from build123d import *

# Parameters (mm, degrees)
F0_W     = 90
F0_H     = 800
F1_DEPTH = 12
F3_D     = 15
F4_SIZE2 = 74.6410161514
F4_SIZE  = 20
F6_D     = 5


with BuildPart() as f1:
    # F0 (on Front) → F1 (new body)
    with BuildSketch(Plane.XZ):
        with Locations((45, -400)):
            Rectangle(F0_W, F0_H)
    extrude(amount=F1_DEPTH)

    # F3 (through all)
    with Locations(Plane.XZ.offset(12)):
        with Locations((45, -35)):
            Hole(F3_D / 2)

    # F4
    f4_edges = [f1.edges().sort_by_distance(p)[0] for p in [
        (90, -6, -800),
    ]]
    f4_side = f1.faces().sort_by_distance((90, -6, -400))[0]
    chamfer(f4_edges, length=F4_SIZE, length2=F4_SIZE2, reference=f4_side)

    # F6 (through all)
    with Locations(Plane.XZ.offset(12)):
        with Locations((40, -380), (40, -540)):
            Hole(F6_D / 2)


solid = f1.part
Verification items for the finished model (mm, model axes). Give positions to 0.01 mm unless a question says otherwise; leave off trailing zeros. Loops run counter-clockwise (first coordinate to the right, second up) from the corner with the lowest first, then second, coordinate; pieces in that order, holes last. Notation, with made-up numbers: (69.25, -37.5) - (87.25, -37.5) arc R14 cw to (87.25, -25.5) - close; hole circle Ø3 at (1, 3). An arc over 180 degrees is marked (long way). Write each question's results on one line, items separated by ' | '.
1) Mould release check, pull along Z, two halves, no side actions. Record for faces 1 (the flat face through (44, 0, -394)), 2 (the cylindrical face through (41.539, -5.916, -41.654)), 3 (the flat face through (52.16, -5.92, -790.14)): pulls with the +Z half, pulls with the -Z half, needs draft (parallel to the pull), parting line crosses it, or undercut.
Solution:
face 1: needs draft | face 2: undercut | face 3: pulls with the -Z half
2) Sectioned sample at A-A on z = -35. Record the boundary of the cut face in (x, y), plus the area to 3 significant figures.
Solution:
outline: (0, -12) - (37.5, -12) - (37.5, 0) - (0, 0) - close; (52.5, -12) - (90, -12) - (90, 0) - (52.5, 0) - close | area: 900 mm2
3) Depth check by flat-ended pin: P1, Ø1, axis at x = 17, y = -1.5, coming from the -Z side. Enter the tip coordinate at first touch or a pass-through.
Solution:
P1: z = -799.69
4) Sectioned sample at B-B on x = 66.5. Record the boundary of the cut face in (y, z).
Solution:
outline: (-12, -786.3) - (0, -786.3) - (0, 0) - (-12, 0) - close
5) Material ranges on L1, parallel to Z at x = 41, y = -9; L2, parallel to Z at x = 38.5, y = -7; L3, parallel to X at y = -8.75, z = -380, recorded low to high. Write a range as from..to.
Solution:
L1: -793.13..-542.29, -537.71..-382.29, -377.71..-41.34, -28.66..0 | L2: -793.8..-542, -538..-382, -378..-38.74, -31.26..0 | L3: 0..37.5, 42.5..90
